For this review, use the dimensioned drawing (mm, ordinates from the lowest corner) and the shaded views. A direction names the side the tool comes from. Coordinates: 2 decimals unless noted, no trailing zeros. Loops run counter-clockwise (first coordinate to the right, second up) from the corner with the lowest first, then second, coordinate; pieces in that order, holes last. Notation, with made-up numbers: (69.5, -24.5) - (81.5, -24.5) arc R10 ccw to (81.5, -19.5) - close; hole circle Ø2 at (72.25, 80.25). An arc over 180 degrees is marked (long way). Use one line per item in the form item = value. Start each with the question number.
(1) Add section D-D (x = 20). State the section outline as (y, z) points.
(2) Add section A-A (x = 43). State the section outline as (y, z) points, plus the area to 3 significant figures.
(3) The part is to be moulded in two halves that separate along Y. For the marked faces 1, 2 and 3, say which applies: pulls with the +Y half, pulls with the -Y half, needs draft (parallel to the pull), parting line crosses it, or undercut.
(4) Clearance check with flat-ended pins moving along their axes: pin 1 Ø3 at (x, z) = (45.5, 7) entering from +Y; pin 2 Ø4.5 at (y, z) = (41.5, 12) entering from -X; pin 3 Ø7 at (y, z) = (40, 6) entering from +X; pin 4 Ø12 at (x, y) = (23.5, 37.5) entering from +Z. State where each tip first meets the part, or that it passes through.
(5) Tool access review of the marked faces 4, 5, 6 and 7: name each direction out of +Z, -Z, +X, -X, +Y, -Y from which nothing blocks a thin tool from reaching the whole face with its end or side.
(6) Add section C-C (y = 27). State the section outline as (x, z) points, plus the area to 3 significant figures.
(7) Add section B-B (y = 39). State the section outline as (x, z) points, plus the area to 3 significant figures.
(8) For L1, parallel to X at y = 4, z = 8; L2, parallel to Y at x = 12.5, z = 8; L3, parallel to X at y = 27, z = 10.75, list the stretches that pass through material, from the lowest coordinate up.
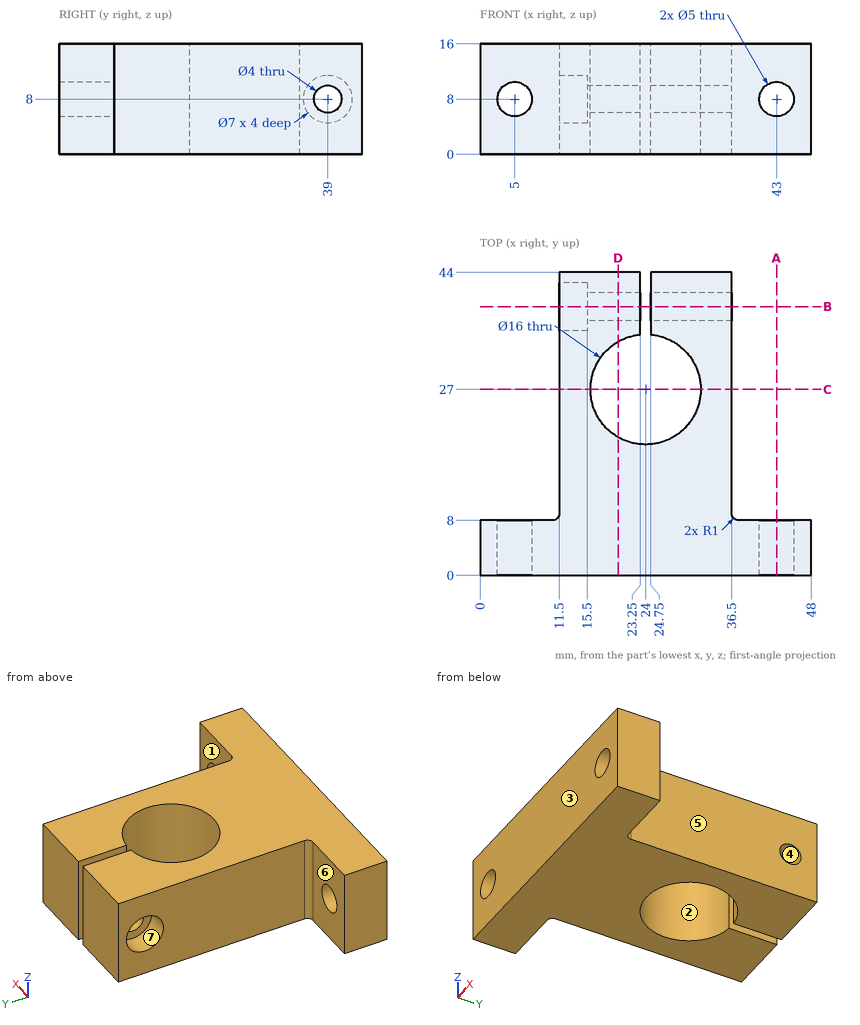
Computed values:
q1.outline = (0, 0) - (20.07, 0) - (20.07, 16) - (0, 16) - close; (33.93, 0) - (44, 0) - (44, 16) - (33.93, 16) - close; hole circle Ø4 at (39, 8)
q2.outline = (0, 0) - (8, 0) - (8, 5.5) - (0, 5.5) - close; (0, 10.5) - (8, 10.5) - (8, 16) - (0, 16) - close
q2.area = 88.0 mm^2
q3.face_1 = pulls with the +Y half
q3.face_2 = undercut
q3.face_3 = pulls with the -Y half
q4.pin_1 = 8
q4.pin_2 = 11.5
q4.pin_3 = 36.5
q4.pin_4 = 16
q5.face_4 = +X, -X
q5.face_5 = +Z, -Z, +X, +Y
q5.face_6 = +Z, -Z, -X, +Y
q5.face_7 = -X
q6.outline = (11.5, 0) - (16, 0) - (16, 16) - (11.5, 16) - close; (32, 0) - (36.5, 0) - (36.5, 16) - (32, 16) - close
q6.area = 144 mm^2
q7.outline = (11.5, 0) - (23.25, 0) - (23.25, 6) - (15.5, 6) - (15.5, 4.5) - (11.5, 4.5) - close; (11.5, 11.5) - (15.5, 11.5) - (15.5, 10) - (23.25, 10) - (23.25, 16) - (11.5, 16) - close; (24.75, 0) - (36.5, 0) - (36.5, 6) - (24.75, 6) - close; (24.75, 10) - (36.5, 10) - (36.5, 16) - (24.75, 16) - close
q7.area = 270 mm^2
q8.L1 = 0 to 2.5, 7.5 to 40.5, 45.5 to 48
q8.L2 = 0 to 35.5, 42.5 to 44
q8.L3 = 11.5 to 16, 32 to 36.5
